```python
from build123d import *

# Parameters (mm, degrees)
SZKIC1_R                    = 1.9
SZKIC1_R_2                  = 46
DODANIE_WYCI_GNI_CIE1_DEPTH = 4


with BuildPart() as part:
    # Szkic1 → Dodanie-wyciągnięcie1 (new body)
    with BuildSketch(Plane.XY):
        with BuildLine():
            add(Edge.make_bspline(
                [(0, 87), (18.224844976, 86.998612649), (32.288902875, 73.536902698), (46.435034931, 63.912342556)],
                knots=[0, 0, 0, 0, 1, 1, 1, 1], degree=3))
            add(Edge.make_bspline(
                [(82.741916918, 26.884478511), (77.108810651, 44.216907368), (59.959930782, 53.43272413), (46.435034931, 63.912342556)],
                knots=[0, 0, 0, 0, 1, 1, 1, 1], degree=3))
            add(Edge.make_bspline(
                [(82.741916918, 26.884478511), (88.372384286, 9.551192223), (79.915570217, -7.984418835), (75.133464787, -24.412342556)],
                knots=[0, 0, 0, 0, 1, 1, 1, 1], degree=3))
            add(Edge.make_bspline(
                [(51.137316949, -70.384478511), (65.88071079, -59.671061018), (69.346178061, -40.513663074), (75.133464787, -24.412342556)],
                knots=[0, 0, 0, 0, 1, 1, 1, 1], degree=3))
            add(Edge.make_bspline(
                [(51.137316949, -70.384478511), (36.39229218, -81.095651222), (17.10163575, -78.471544919), (0, -79)],
                knots=[0, 0, 0, 0, 1, 1, 1, 1], degree=3))
            add(Edge.make_bspline(
                [(-51.137316949, -70.384478511), (-36.39229218, -81.095651222), (-17.10163575, -78.471544919), (0, -79)],
                knots=[0, 0, 0, 0, 1, 1, 1, 1], degree=3))
            add(Edge.make_bspline(
                [(-51.137316949, -70.384478511), (-65.88071079, -59.671061018), (-69.346178061, -40.513663074), (-75.133464787, -24.412342556)],
                knots=[0, 0, 0, 0, 1, 1, 1, 1], degree=3))
            add(Edge.make_bspline(
                [(-82.741916918, 26.884478511), (-88.372384286, 9.551192223), (-79.915570217, -7.984418835), (-75.133464787, -24.412342556)],
                knots=[0, 0, 0, 0, 1, 1, 1, 1], degree=3))
            add(Edge.make_bspline(
                [(-82.741916918, 26.884478511), (-77.108810651, 44.216907368), (-59.959930782, 53.43272413), (-46.435034931, 63.912342556)],
                knots=[0, 0, 0, 0, 1, 1, 1, 1], degree=3))
            add(Edge.make_bspline(
                [(0, 87), (-18.224844976, 86.998612649), (-32.288902875, 73.536902698), (-46.435034931, 63.912342556)],
                knots=[0, 0, 0, 0, 1, 1, 1, 1], degree=3))
        make_face()
        with Locations((0, 79)):
            Circle(SZKIC1_R, mode=Mode.SUBTRACT)
        with Locations((75.133464787, 24.412342556)):
            Circle(SZKIC1_R, mode=Mode.SUBTRACT)
        with Locations((46.435034931, -63.912342556)):
            Circle(SZKIC1_R, mode=Mode.SUBTRACT)
        with Locations((-46.435034931, -63.912342556)):
            Circle(SZKIC1_R, mode=Mode.SUBTRACT)
        with Locations((-75.133464787, 24.412342556)):
            Circle(SZKIC1_R, mode=Mode.SUBTRACT)
        Circle(SZKIC1_R_2, mode=Mode.SUBTRACT)
        with Locations((35.561007764, 48.94552816)):
            Circle(SZKIC1_R, mode=Mode.SUBTRACT)
        with Locations((57.538919236, -18.69552816)):
            Circle(SZKIC1_R, mode=Mode.SUBTRACT)
        with Locations((0, -60.5)):
            Circle(SZKIC1_R, mode=Mode.SUBTRACT)
        with Locations((-57.538919236, -18.69552816)):
            Circle(SZKIC1_R, mode=Mode.SUBTRACT)
        with Locations((-35.561007764, 48.94552816)):
            Circle(SZKIC1_R, mode=Mode.SUBTRACT)
    extrude(amount=DODANIE_WYCI_GNI_CIE1_DEPTH)


solid = part.part
```
Input: part model. Units: mm. Frame: model coordinates. Coordinates: 2 decimals unless noted, no trailing zeros. Answer in a Markdown table with one row per item.
(1) Pin query (flat end, axial travel): P1, Ø1.5, axis at y = 16.5, z = 2, coming from the +X side; P2, Ø1.5, axis at x = 50.5, z = 1, coming from the -Y side. Return the tip coordinate at first contact, or that it passes through.
Model answer:
| item | result |
|---|---|
| P1 | stops at x = 84.6 |
| P2 | stops at y = -71.34 |
(2) Cut plane A-A on z = 0.95. Count the separate pieces of the cut face and the enclosed holes in it, plus the area to 3 significant figures.
Model answer:
| item | result |
|---|---|
| separate pieces | 1 |
| enclosed holes | 11 |
| area | 14,800 mm² |
(3) Mould query, pull axis Y, two halves, no side actions, for faces 1 (the face through (-33.75, 49.52, 1.97)), 2 (the face through (41, 23, 4)). Classes: pulls with the +Y half, pulls with the -Y half, needs draft (parallel to the pull), parting line crosses it, or undercut.
Model answer:
| item | result |
|---|---|
| face 1 | undercut |
| face 2 | needs draft |
(4) Material intervals for L1, parallel to Y at x = 35, z = 3.2; L2, parallel to X at y = 0.5, z = 2.45; L3, parallel to X at y = 48.5, z = 1.15, sorted ascending. Write a range as from..to.
Model answer:
| item | result |
|---|---|
| L1 | y = -77.29..-29.85, 29.85..47.13, 50.76..72.14 |
| L2 | x = -82.75..-46, 46..82.75 |
| L3 | x = -66.93..-37.41, -33.71..33.71, 37.41..66.93 |
